from build123d import *

# Parameters (mm, degrees)
F1_DEPTH = 175
F2_R     = 2.1
F3_DEPTH = 25
F4_DEPTH = 25
F5_DEPTH = 5
F6_DEPTH = 5


with BuildPart() as f1:
    # F0 (on Front) → F1 (new body)
    with BuildSketch(Plane.XZ):
        Polygon((4.5, 4), (11, 10), (-11, 10), (-4.5, 4), (0, 4), align=None)
        Polygon((11, 10), (21.9141976312, 10), (21.9141976312, 12.2224409133), (-21.9141976312, 12.2224409133), (-21.9141976312, 10), (-11, 10), align=None)
    extrude(amount=F1_DEPTH)

    # F2 (on face) → F3 (cut)
    with BuildSketch(Plane(origin=(0, 0, 4), x_dir=(1, 0, 0), z_dir=(0, 0, -1))):
        with Locations((0, 136.6154402494)):
            Circle(F2_R)
    extrude(amount=-F3_DEPTH, mode=Mode.SUBTRACT)

    # F2 (on face) → F4 (cut)
    with BuildSketch(Plane(origin=(0, 0, 4), x_dir=(1, 0, 0), z_dir=(0, 0, -1))):
        with Locations((0, 30.1199369133)):
            Circle(F2_R)
    extrude(amount=-F4_DEPTH, mode=Mode.SUBTRACT)

    # F2 (on face) → F5 (cut)
    with BuildSketch(Plane(origin=(0, 0, 4), x_dir=(1, 0, 0), z_dir=(0, 0, -1))):
        with BuildLine():
            ThreePointArc((4.5, 25.4295211534), (5.9791303716, 27.5704271565), (6.5, 30.1199369133))
            ThreePointArc((6.5, 30.1199369133), (5.9791303716, 32.66944667), (4.5, 34.8103526731))
            Line((4.5, 34.8103526731), (4.5, 25.4295211534))
        make_face()
        with BuildLine():
            Line((4.5, 25.4295211534), (4.5, 34.8103526731))
            ThreePointArc((4.5, 34.8103526731), (0, 36.6199369133), (-4.5, 34.8103526731))
            Line((-4.5, 34.8103526731), (-4.5, 25.4295211534))
            ThreePointArc((-4.5, 25.4295211534), (0, 23.6199369133), (4.5, 25.4295211534))
        make_face()
        with Locations((0, 30.1199369133)):
            Circle(F2_R, mode=Mode.SUBTRACT)
        with BuildLine():
            Line((-4.5, 25.4295211534), (-4.5, 34.8103526731))
            ThreePointArc((-4.5, 34.8103526731), (-6.5, 30.1199369133), (-4.5, 25.4295211534))
        make_face()
        with BuildLine():
            Line((4.5, 141.3058560093), (4.5, 131.9250244896))
            ThreePointArc((4.5, 131.9250244896), (5.9791303716, 134.0659304926), (6.5, 136.6154402494))
            ThreePointArc((6.5, 136.6154402494), (5.9791303716, 139.1649500062), (4.5, 141.3058560093))
        make_face()
    extrude(amount=-F5_DEPTH, mode=Mode.SUBTRACT)

    # F2 (on face) → F6 (cut)
    with BuildSketch(Plane(origin=(0, 0, 4), x_dir=(1, 0, 0), z_dir=(0, 0, -1))):
        with BuildLine():
            ThreePointArc((-4.5, 141.3058560093), (-6.5, 136.6154402494), (-4.5, 131.9250244896))
            Line((-4.5, 131.9250244896), (-4.5, 141.3058560093))
        make_face()
        with BuildLine():
            ThreePointArc((-4.5, 131.9250244896), (0, 130.1154402494), (4.5, 131.9250244896))
            Line((4.5, 131.9250244896), (4.5, 141.3058560093))
            ThreePointArc((4.5, 141.3058560093), (0, 143.1154402494), (-4.5, 141.3058560093))
            Line((-4.5, 141.3058560093), (-4.5, 131.9250244896))
        make_face()
        with Locations((0, 136.6154402494)):
            Circle(F2_R, mode=Mode.SUBTRACT)
    extrude(amount=-F6_DEPTH, mode=Mode.SUBTRACT)


solid = f1.part
The listing builds one solid part. Answer for the finished solid, in the listing's coordinates (mm). A direction names the side the tool comes from. Round coordinates to 2 decimals unless told otherwise and drop trailing zeros. Order: outer loops, then holes, each group sorted by start corner. A loop starts at its lowest first (then second) coordinate and runs counter-clockwise, first axis right, second up. Notation, with made-up numbers: (-21, 46) -> (-12, 46) arc R21 cw to (-12, 62) -> close; hole circle Ø1 at (48, -7.5). An arc over 180 degrees is marked (long way). Write each question's results on one line, items separated by ' | '. Start each with the question number.
Q1. Each of these flat-tipped pins is pushed along its axis until it touches: pin 1 (6.5 mm diameter, centred on x = 0, y = -136.62, fed in from +Z); pin 2 (12 mm diameter, centred on x = -16, y = -91, fed in from -Z); pin 3 (4 mm diameter, centred on x = 0, y = -30.12, fed in from -Z); pin 4 (5.5 mm diameter, centred on x = 19, y = -129.5, fed in from -Z). Where does it stop, or does it pass through?
Q2. Find section A-A (x = 0). Determine the outline of the cut face in (y, z), then the cut area to 3 significant figures.
Q3. The mould has two halves that part along X. Classify faces 1 (the flat face through (-7.795, -86.275, 7.042)), 2 (the flat face through (0, -83, 4)), 3 (the flat face through (-2, -32, 9)): pulls with the +X half, pulls with the -X half, needs draft (parallel to the pull), parting line crosses it, or undercut.
Q4. Straight lines are drawn through the part: probe 1 along Y at (x, z) = (0, 11); probe 2 along Y at (x, z) = (-1.5, 8.25); probe 3 along Z at (x, y) = (-11, -71). For each, find the intervals that lie inside material, in ascending order. Write a range as from..to.
Q5. Which of the six approach directions +Z, -Z, +X, -X, +Y, -Y give full straight-line access (tool end or side, diameter ignored) to faces 4 (the flat face through (-2, -138, 9)), 5 (the flat face through (-17, -86, 10)), 6 (the flat face through (16, -86, 10))?
Q6. Find section B-B (y = -88). Determine the outline of the cut face in (x, z), then the cut area to 3 significant figures.
Q7. Find section C-C (x = 18). Determine the outline of the cut face in (y, z), then the cut area to 3 significant figures.
Worked answers:
1) pin 1: stops at z = 12.22 | pin 2: stops at z = 9.08 | pin 3: passes through | pin 4: stops at z = 10
2) outline: (-175, 4) -> (-143.12, 4) -> (-143.12, 9) -> (-138.72, 9) -> (-138.72, 12.22) -> (-175, 12.22) -> close; (-134.52, 9) -> (-130.12, 9) -> (-130.12, 4) -> (-36.62, 4) -> (-36.62, 9) -> (-32.22, 9) -> (-32.22, 12.22) -> (-134.52, 12.22) -> close; (-28.02, 9) -> (-23.62, 9) -> (-23.62, 4) -> (0, 4) -> (0, 12.22) -> (-28.02, 12.22) -> close | area: 1,280 mm2
3) face 1: pulls with the -X half | face 2: needs draft | face 3: undercut
4) probe 1: y = -175..-138.72, -134.52..-32.22, -28.02..0 | probe 2: y = -175..-142.94, -130.29..-36.44, -23.8..0 | probe 3: z = 10..12.22
5) face 4: -Z | face 5: -Z, -X, +Y, -Y | face 6: -Z, +X, +Y, -Y
6) outline: (-21.91, 10) -> (-11, 10) -> (-4.5, 4) -> (4.5, 4) -> (11, 10) -> (21.91, 10) -> (21.91, 12.22) -> (-21.91, 12.22) -> close | area: 190 mm2
7) outline: (-175, 10) -> (0, 10) -> (0, 12.22) -> (-175, 12.22) -> close | area: 389 mm2
